```python
from build123d import *

# Parameters (mm, degrees)
PAD004_DEPTH    = 51
POCKET008_DEPTH = 49
SKETCH014_R     = 2.5
POCKET009_DEPTH = 111.501
SKETCH015_R     = 6
POCKET010_DEPTH = 27
PAD005_DEPTH    = 2
SKETCH017_R     = 2.5
POCKET011_DEPTH = 5


with BuildPart() as part:
    # Sketch012 → Pad004 (new body)
    with BuildSketch(Plane.XY):
        Polygon((40, 50), (-66, 15), (-69.5, 10), (-66, 0), (0, 0), (20, -20), (42, -20), (42, 50), align=None)
    extrude(amount=PAD004_DEPTH)

    # Sketch013 (on Face10 of Pad004) → Pocket008 (cut)
    with BuildSketch(Plane.XY.offset(51)):
        Polygon((40, 50), (-66, 15), (-66, 10), (40, 10), align=None)
    extrude(amount=-POCKET008_DEPTH, mode=Mode.SUBTRACT)

    # Sketch014 (on Face10 of Pocket008) → Pocket009 (cut, through all)
    with BuildSketch(Plane.YZ.offset(42)):
        with Locations((-6.5, 25.5)):
            Circle(SKETCH014_R)
    extrude(amount=-POCKET009_DEPTH, mode=Mode.SUBTRACT)

    # Sketch015 → Pocket010 (cut)
    with BuildSketch(Plane.YZ):
        with Locations((-6.5, 25.5)):
            Circle(SKETCH015_R)
    extrude(amount=POCKET010_DEPTH, mode=Mode.SUBTRACT)

    # Sketch016 → Pad005 (join)
    with BuildSketch(Plane.XY):
        Polygon((53.464466, 50), (42, 50), (42, 35), (53.464466, 35), (57, 38.535534), (57, 46.464466), align=None)
    extrude(amount=PAD005_DEPTH)

    # Sketch017 (on Face19 of Pad005) → Pocket011 (cut)
    with BuildSketch(Plane.XY.offset(2)):
        with Locations((49.5, 42.5)):
            Circle(SKETCH017_R)
    extrude(amount=-POCKET011_DEPTH, mode=Mode.SUBTRACT)


with BuildPart() as part_1:
    # Body001 placement: moved
    add(part.part.moved(Location((-99, 14, -66.5))))


solid = part_1.part
```
For this review, take the finished solid that the model builds, in its own axes (mm). A direction names the side the tool comes from. Give positions to 0.01 mm unless a question says otherwise; leave off trailing zeros. Write each loop counter-clockwise with the first axis right and the second up, starting at its lowest first coordinate (ties: lowest second). Pieces come first, ordered by that corner, then holes.
Item 1: The part is to be moulded in two halves that separate along Y. For faces 6 (the face through (-64.4, 6.96, -43.44)), 7 (the face through (-111.258, 46.745, -65.514)), 8 (the face through (-166.774, 19.07, -41.357)), say which applies: +Y half, -Y half, draft (parallel to the pull), parting line (faces both ways), or undercut.
Item 2: Take a section at A-A (z = -41). Give the boundary of the cut face in (x, y).
Item 3: Take a section at D-D (y = 43). Give the boundary of the cut face in (x, z).
Item 4: Take a section at B-B (x = -49.5). Give the boundary of the cut face in (y, z), and give its area (3 significant figures).
Item 5: Wall thickness on probe 1 along Y at (x, z) = (-49.5, -65.7); probe 2 along Z at (x, y) = (-66.5, 7.5); probe 3 along Z at (x, y) = (-90.75, 7.5): over which ranges is each line inside the solid? List them lowest first.
Item 6: Take a section at C-C (y = 7.5). Give the boundary of the cut face in (x, z).
Item 7: Machinability: for faces 1 (the face through (-82.491, 13.223, -39.198)), 2 (the face through (-53, 57, -64.5)), 3 (the face through (-101, 40, -64.5)), 4 (the face through (-132, 14, -41)), 5 (the face through (-47.19, 55.54, -65.49)), which of the approach directions +Z, -Z, +X, -X, +Y, -Y give a long, thin tool a straight path to every point of the face, cutting with its end or side? Answer none if there is none.
Item 8: Insertion check: P1, Ø4.5, axis at x = -49.5, y = 56.5, coming from the +Z side; P2, Ø3, axis at y = 12, z = -60.5, coming from the -X side; P3, Ø20, axis at x = -96.5, y = 38, coming from the +Z side; P4, Ø7, axis at y = 7.5, z = -41, coming from the +X side. Each pin has a flat end and moves straight along its axis. Give the tip position at first contact, or say it passes through.
Established:
1. face 6: undercut
1. face 7: +Y half
1. face 8: -Y half
2. outline: (-168.5, 24) - (-165, 14) - (-99, 14) - (-98.5, 13.5) - (-72, 13.5) - (-72, 10) - (-57, 10) - (-57, 64) - (-59, 64) - (-59, 24) - (-165, 24) - (-165, 29) - close; (-86.5, 1.5) - (-79, -6) - (-57, -6) - (-57, 5) - (-72, 5) - (-72, 1.5) - close
3. outline: (-122.6, -66.5) - (-57, -66.5) - (-57, -15.5) - (-59, -15.5) - (-59, -64.5) - (-122.6, -64.5) - close
4. outline: (49, -66.5) - (54, -66.5) - (54, -64.5) - (49, -64.5) - close; (59, -66.5) - (64, -66.5) - (64, -64.5) - (59, -64.5) - close
4. area: 20.0 mm2
5. probe 1: y = 49 to 54, 59 to 64
5. probe 2: z = -66.5 to -43.5, -38.5 to -15.5
5. probe 3: z = -66.5 to -47, -35 to -15.5
6. outline: (-92.5, -66.5) - (-57, -66.5) - (-57, -43.5) - (-72, -43.5) - (-72, -47) - (-92.5, -47) - close; (-92.5, -35) - (-72, -35) - (-72, -38.5) - (-57, -38.5) - (-57, -15.5) - (-92.5, -15.5) - close
7. face 1: -X
7. face 2: +Z, +X, +Y, -Y
7. face 3: +Z, +Y
7. face 4: +Z, -Z, -X, -Y
7. face 5: +Z, -Z
8. P1: passes through
8. P2: stops at x = -98.5
8. P3: stops at z = -64.5
8. P4: stops at x = -57
